For this review, use the dimensioned drawing (mm, ordinates from the lowest corner) and the shaded views. A direction names the side the tool comes from. Coordinates: 2 decimals unless noted, no trailing zeros. Order: outer loops, then holes, each group sorted by start corner. A loop starts at its lowest first (then second) coordinate and runs counter-clockwise, first axis right, second up. Notation, with made-up numbers: M -21.75,74.5 L -2.75,74.5 A16 ccw -2.75,84.5 Z; hole C 84.25,58 d4. An arc over 180 degrees is marked long. Use one line per item in the form item = value. Start each with the question number.
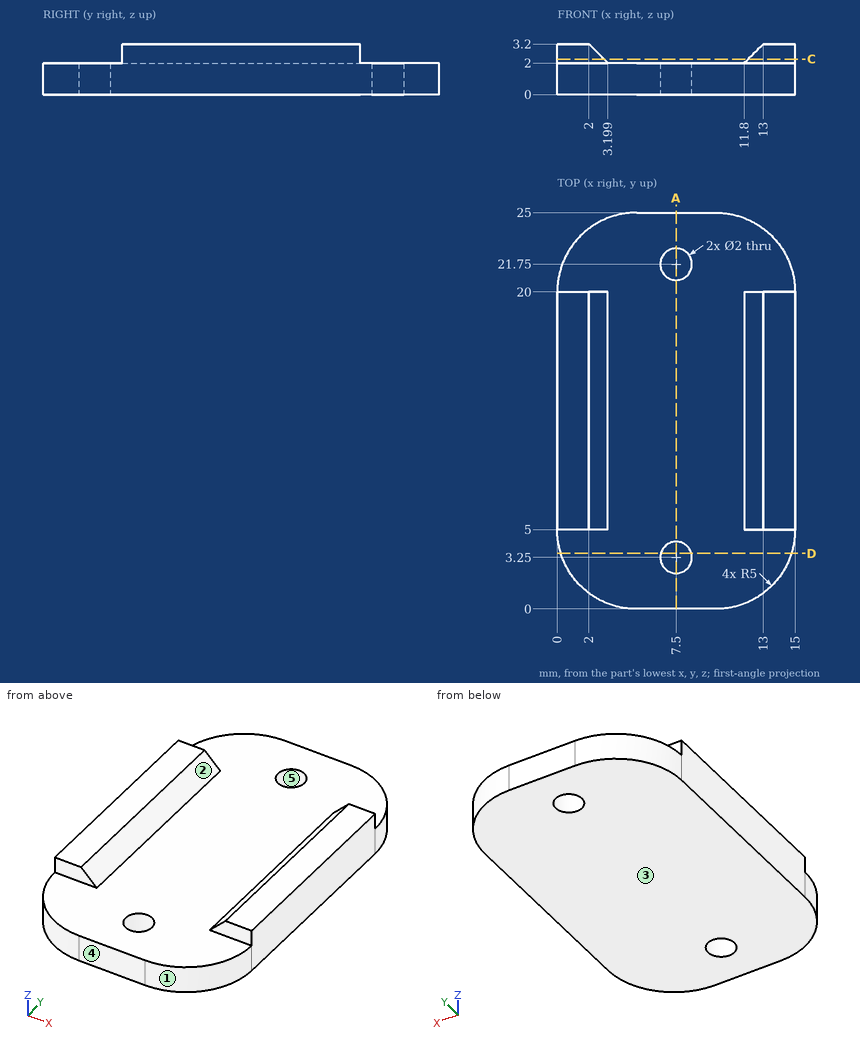
1. The part is to be moulded in two halves that separate along Y. For the marked faces 3, 4 and 5, say which applies: pulls with the +Y half, pulls with the -Y half, needs draft (parallel to the pull), parting line crosses it, or undercut.
2. For pin 1 Ø2.5 at (x, y) = (7.5, 3.25) entering from +Z; pin 2 Ø1.5 at (x, z) = (13, 1.5) entering from -Y (1 decimal); pin 3 Ø1.3 at (x, z) = (14, 2.5) entering from -Y (1 decimal), all flat-tipped, find the tip position at first contact; note any pin that passes through.
3. Consider section C-C, the plane z = 2.25. Write out the cut boundary in (x, y).
4. Consider section A-A, the plane x = 7.5. Write out the cut boundary in (y, z).
5. Consider section D-D, the plane y = 3.5. Write out the cut boundary in (x, z), plus the area to 3 significant figures.
6. Tool access review of the marked faces 1 and 2: name each direction out of +Z, -Z, +X, -X, +Y, -Y from which nothing blocks a thin tool from reaching the whole face with its end or side.
7. To check wall thickness, follow line 1 (Y direction, x = 7.5, z = 0.75); line 2 (Z direction, x = 9.75, y = 11); line 3 (Y direction, x = 12.5, z = 1). State the ranges of each line that lie inside material, in increasing order.
Answers follow:
q1.face_3 = needs draft
q1.face_4 = pulls with the -Y half
q1.face_5 = undercut
q2.pin_1 = 2
q2.pin_2 = 0.5
q2.pin_3 = 1.5
q3.outline = M 0,5 L 2.95,5 L 2.95,20 L 0,20 Z; M 12.05,5 L 15,5 L 15,20 L 12.05,20 Z
q4.outline = M 0,0 L 2.25,0 L 2.25,2 L 0,2 Z; M 4.25,0 L 20.75,0 L 20.75,2 L 4.25,2 Z; M 22.75,0 L 25,0 L 25,2 L 22.75,2 Z
q5.outline = M 0.23,0 L 6.53,0 L 6.53,2 L 0.23,2 Z; M 8.47,0 L 14.77,0 L 14.77,2 L 8.47,2 Z
q5.area = 25.2 mm²
q6.face_1 = +Z, -Z, +X, -Y
q6.face_2 = +Z, +Y, -Y
q7.line_1 = 0 to 2.25, 4.25 to 20.75, 22.75 to 25
q7.line_2 = 0 to 2
q7.line_3 = 0.67 to 24.33
